Solid Edge part; units mm, degrees
sketch "Sketch1" plane through (0, 0, 0) normal (0, -1, 0) x (1, 0, 0)
  line L0 (33.7037, 66.6239) -> (103.7037, 66.6239)
  line L1 (103.7037, 66.6239) -> (103.7037, 26.6239)
  line L2 (103.7037, 26.6239) -> (33.7037, 26.6239)
  line L3 (33.7037, 26.6239) -> (33.7037, 66.6239)
  dimension "D1" = 33.7037
  dimension "D2" = 103.7037
  dimension "D3" = 103.7037
  dimension "D4" = 33.7037
extrude "Protrusion1" add sketch "Sketch1" against normal blind 15
sketch "Sketch2" plane through (68.7037, 0, 46.6239) normal (0, -1, 0) x (1, 0, 0)
  circle A0 centre (0, 10) radius 5.5
extrude "ExtrudedCutout_1" cut sketch "Sketch2" against normal blind 12
sketch "Sketch3" plane through (103.7037, 7.5, 46.6239) normal (1, 0, 0) x (0, 1, 0)
  line L0 (-7.5, 12.6) -> (-1.5, 12.6)
  arc A0 (-1.5, 12.6) -> (-1.5, 7.4) centre (-1.5, 10) cw
  line L1 (-1.5, 7.4) -> (-7.5, 7.4)
  line L2 (-7.5, 7.4) -> (-7.5, 12.6)
  dimension "D1" = 7.5
extrude "ExtrudedCutout_4" cut sketch "Sketch3" against normal blind 15
sketch "Sketch4" plane through (88.7037, 4.3, 55.6239) normal (1, 0, 0) x (0, 1, 0)
  line L0 (-4.3, 6) -> (1.7, 6)
  arc A0 (1.7, 6) -> (1.7, -5) centre (1.7, 0.5) cw
  line L1 (1.7, -5) -> (-4.3, -5)
  line L2 (-4.3, -5) -> (-4.3, 6)
  dimension "D1" = 4.3
extrude "ExtrudedCutout_5" cut sketch "Sketch4" against normal blind 15
sketch "Sketch5" plane through (33.7037, 7.5, 46.6239) normal (-1, 0, 0) x (0, -1, 0)
  line L0 (7.5, 12.6) -> (1.5, 12.6)
  arc A0 (1.5, 12.6) -> (1.5, 7.4) centre (1.5, 10) ccw
  line L1 (1.5, 7.4) -> (7.5, 7.4)
  line L2 (7.5, 7.4) -> (7.5, 12.6)
  dimension "D1" = 7.5
  dimension "D2" = 7.5
extrude "ExtrudedCutout_6" cut sketch "Sketch5" against normal blind 15
sketch "Sketch6" plane through (48.7037, 4.3, 56.6239) normal (-1, 0, 0) x (0, -1, 0)
  line L0 (4.3, 5.5) -> (-1.7, 5.5)
  arc A0 (-1.7, 5.5) -> (-1.7, -5.5) centre (-1.7, 0) ccw
  line L1 (-1.7, -5.5) -> (4.3, -5.5)
  line L2 (4.3, -5.5) -> (4.3, 5.5)
  dimension "D1" = 4.3
  dimension "D2" = 4.3
extrude "ExtrudedCutout_7" cut sketch "Sketch6" against normal blind 9
sketch "Sketch7" plane through (57.7037, 5.75, 56.6239) normal (-1, 0, 0) x (0, -1, 0)
  line L0 (5.75, 3.9) -> (-0.25, 3.9)
  arc A0 (-0.25, 3.9) -> (-0.0606, -4.0955) centre (-0.25, -0.1) ccw
  line L1 (-0.0606, -4.0955) -> (5.75, -4.0955)
  line L2 (5.75, -4.0955) -> (5.75, 3.9)
  dimension "D1" = 5.75
  dimension "D2" = 5.75
extrude "Cutout1" cut sketch "Sketch7" against normal up to next
sketch "Sketch8" plane through (68.7037, 7.5, 26.6239) normal (0, 0, -1) x (1, 0, 0)
  line L0 (-6, 7.5) -> (-6, 1.5)
  arc A0 (-6, 1.5) -> (6, 1.5) centre (0, 1.5) ccw
  line L1 (6, 1.5) -> (6, 7.5)
  line L2 (6, 7.5) -> (-6, 7.5)
  dimension "D1" = 6
extrude "ExtrudedCutout_9" cut sketch "Sketch8" against normal blind 13
sketch "Sketch9" plane through (68.7037, 5.75, 39.6239) normal (0, 0, -1) x (1, 0, 0)
  line L0 (-2.4391, 5.75) -> (-2.4391, -0.25)
  arc A0 (-2.4391, -0.25) -> (5.5609, -0.25) centre (1.5609, -0.25) ccw
  line L1 (5.5609, -0.25) -> (5.5609, 5.75)
  line L2 (5.5609, 5.75) -> (-2.4391, 5.75)
  dimension "D1" = 2.4391
extrude "Cutout2" cut sketch "Sketch9" against normal up to next
CAD build for the part. Positions are in the model's coordinates, mm. A direction names the side the tool comes from. Coordinates: 2 decimals unless noted, no trailing zeros. Order: outer loops, then holes, each group sorted by start corner. A loop starts at its lowest first (then second) coordinate and runs counter-clockwise, first axis right, second up. Notation, with made-up numbers: (19.5, -20) -> (31.5, -20) arc R25 cw to (31.5, 16) -> close; hole circle Ø2 at (77, 28.5). An arc over 180 degrees is marked (long way). Use one line per item in the form item = value. Start each with the question number.
1) Pull direction X, two halves, no side cores. Call faces 4 (the flat face through (69, 15, 46)), 5 (the flat face through (82, 3, 50.624)), 6 (the flat face through (33.704, 7, 46)): +X half, -X half, draft (parallel to the pull), parting line (faces both ways), or undercut.
2) Band-saw the part on B-B on x = 41.5. Give the cut face in (y, z).
3) Band-saw the part on C-C on z = 35. Give the cut face in (x, y), then the cut area to 3 significant figures.
4) Drill centre lines: L1, parallel to X at y = 4.5, z = 38.5; L2, parallel to X at y = 1.75, z = 52; L3, parallel to X at y = 1, z = 43. Where is each one in solid material? Low to high. Write a range as [from, to].
5) Band-saw the part on A-A on y = 3.25. State how many separate pieces and enclosed holes the cut face has, then the cut area to 3 significant figures.
6) Band-saw the part on D-D on z = 57.5. Give the cut face in (x, y).
7) Tool access for faces 1 (the flat face through (62.704, 3, 33)), 2 (the flat face through (68, 7, 66.624)), 3 (the cylindrical face through (81.3, 11.5, 56)): list every direction of +Z, -Z, +X, -X, +Y, -Y with a clear straight run to the whole face (end or side of a thin tool).
Entries:
q1.face_4 = draft
q1.face_5 = undercut
q1.face_6 = -X half
q2.outline = (0, 26.62) -> (15, 26.62) -> (15, 66.62) -> (0, 66.62) -> (0, 59.22) -> (6, 59.22) arc R2.6 cw to (6, 54.02) -> (0, 54.02) -> close
q3.outline = (33.7, 0) -> (62.7, 0) -> (62.7, 6) arc R6 cw to (74.7, 6) -> (74.7, 0) -> (103.7, 0) -> (103.7, 15) -> (33.7, 15) -> close
q3.area = 921 mm2
q4.L1 = [33.7, 62.7], [74.7, 103.7]
q4.L2 = [33.7, 48.7], [57.7, 65.73], [88.7, 103.7]
q4.L3 = [33.7, 66.26], [74.26, 103.7]
q5.separate_pieces = 3
q5.enclosed_holes = 0
q5.area = 1,990 mm2
q6.outline = (33.7, 8.45) -> (48.7, 8.45) -> (48.7, 11.43) -> (57.7, 11.43) -> (57.7, 9.88) -> (63.27, 9.88) -> (63.27, 12) -> (74.13, 12) -> (74.13, 11.33) -> (88.7, 11.33) -> (88.7, 8.45) -> (103.7, 8.45) -> (103.7, 15) -> (33.7, 15) -> close
q7.face_1 = -Z, -Y
q7.face_2 = +Z, +X, -X, +Y, -Y
q7.face_3 = -Y
